from build123d import *

# Parameters (mm, degrees)
SKETCH1_R               = 45.95
BOSS_EXTRUDE1_DEPTH     = 3
SKETCH2_R               = 45.95
SKETCH2_R_2             = 40.95
BOSS_EXTRUDE2_DEPTH     = 22.4
SKETCH11_R              = 1.5
CUT_EXTRUDE1_DEPTH      = 46.95
CUT_EXTRUDE1_DEPTH_BACK = 46.95
SKETCH12_R              = 45.95
SKETCH12_R_2            = 40.95
BOSS_EXTRUDE3_DEPTH     = 25.4
SKETCH14_R              = 1.5
CUT_EXTRUDE2_DEPTH      = 46.95000011
CUT_EXTRUDE2_DEPTH_BACK = 46.95000011
SKETCH17_R              = 1.5
CUT_EXTRUDE4_DEPTH      = 10
SKETCH15_R              = 4
CUT_EXTRUDE6_DEPTH      = 10


with BuildPart() as part:
    # Sketch1 → Boss-Extrude1 (new body)
    with BuildSketch(Plane(origin=(0, 0, 0), x_dir=(1, 0, 0), z_dir=(0, 1, 0))):
        Circle(SKETCH1_R)
    extrude(amount=BOSS_EXTRUDE1_DEPTH)

    # Sketch2 → Boss-Extrude2 (add)
    with BuildSketch(Plane(origin=(0, 3, 0), x_dir=(1, 0, 0), z_dir=(0, 1, 0))):
        Circle(SKETCH2_R)
        Circle(SKETCH2_R_2, mode=Mode.SUBTRACT)
    extrude(amount=BOSS_EXTRUDE2_DEPTH)

    # Sketch11 → Cut-Extrude1 (cut, two sides)
    with BuildSketch(Plane.XY) as cut_extrude1_sk:
        with Locations((0, 13.9)):
            Circle(SKETCH11_R)
        with Locations((0, -13.9)):
            Circle(SKETCH11_R)
    extrude(amount=CUT_EXTRUDE1_DEPTH, mode=Mode.SUBTRACT)
    extrude(cut_extrude1_sk.sketch, amount=-CUT_EXTRUDE1_DEPTH_BACK, mode=Mode.SUBTRACT)

    # Sketch12 → Boss-Extrude3 (add)
    with BuildSketch(Plane(origin=(0, 25.4, 0), x_dir=(1, 0, 0), z_dir=(0, 1, 0))):
        Circle(SKETCH12_R)
        Circle(SKETCH12_R_2, mode=Mode.SUBTRACT)
    extrude(amount=BOSS_EXTRUDE3_DEPTH)

    # Sketch14 → Cut-Extrude2 (cut, two sides)
    with BuildSketch(Plane.XY) as cut_extrude2_sk:
        with Locations((0, 36.9)):
            Circle(SKETCH14_R)
    extrude(amount=CUT_EXTRUDE2_DEPTH, mode=Mode.SUBTRACT)
    extrude(cut_extrude2_sk.sketch, amount=-CUT_EXTRUDE2_DEPTH_BACK, mode=Mode.SUBTRACT)

    # Sketch17 → Cut-Extrude4 (cut)
    with BuildSketch(Plane(origin=(0, 3, 0), x_dir=(1, 0, 0), z_dir=(0, 1, 0))):
        with Locations((0, 9.5)):
            Circle(SKETCH17_R)
        with Locations((8.227241336, 4.75)):
            Circle(SKETCH17_R)
        with Locations((8.227241336, -4.75)):
            Circle(SKETCH17_R)
        with Locations((0, -9.5)):
            Circle(SKETCH17_R)
        with Locations((-8.227241336, -4.75)):
            Circle(SKETCH17_R)
        with Locations((-8.227241336, 4.75)):
            Circle(SKETCH17_R)
    extrude(amount=-CUT_EXTRUDE4_DEPTH, mode=Mode.SUBTRACT)

    # Sketch15 → Cut-Extrude6 (cut)
    with BuildSketch(Plane(origin=(0, 3, 0), x_dir=(1, 0, 0), z_dir=(0, 1, 0))):
        Circle(SKETCH15_R)
    extrude(amount=-CUT_EXTRUDE6_DEPTH, mode=Mode.SUBTRACT)


solid = part.part
Source: CAD feature listing. Evaluate the final solid. Frame: model axes, mm. A direction names the side the tool comes from. Give positions to 0.01 mm unless a question says otherwise; leave off trailing zeros. Order: outer loops, then holes, each group sorted by start corner. A loop starts at its lowest first (then second) coordinate and runs counter-clockwise, first axis right, second up. Notation, with made-up numbers: (-14, -26.5) -> (27, -26.5) arc R8 cw to (27, -15.5) -> close; hole circle Ø7 at (72.25, -33). An arc over 180 degrees is marked (long way). Use a Markdown table: item, result.
1) Section query A-A, the plane z = 0. Return the cut outline in (x, y).
Answer list:
| item | result |
|---|---|
| outline | (-45.95, 0) -> (-4, 0) -> (-4, 3) -> (-40.95, 3) -> (-40.95, 50.8) -> (-45.95, 50.8) -> close; (4, 0) -> (45.95, 0) -> (45.95, 50.8) -> (40.95, 50.8) -> (40.95, 3) -> (4, 3) -> close |
2) Ray query, line 1 along Z through (x, y) = (0, 2.25); line 2 along X through (y, z) = (19, 0); line 3 along Z through (x, y) = (-1.5, 32.5). Return the intervals inside material, ascending. Write a range as [from, to].
Answer list:
| item | result |
|---|---|
| line 1 | [-45.95, -11], [-8, -4], [4, 8], [11, 45.95] |
| line 2 | [-45.95, -40.95], [40.95, 45.95] |
| line 3 | [-45.93, -40.92], [40.92, 45.93] |
3) Mould query, pull axis Z, two halves, no side actions, for faces 1 (the cylindrical face through (9.613, 1.521, -4.175)), 2 (the flat face through (10, 0, -1)), 3 (the cylindrical face through (-9.961, 25.044, 44.857)). Classes: +Z half, -Z half, draft (parallel to the pull), parting line (faces both ways), or undercut.
Answer list:
| item | result |
|---|---|
| face 1 | undercut |
| face 2 | draft |
| face 3 | parting line |
4) Section query D-D, the plane z = -20.5. Return the cut outline in (x, y), then the cut area to 3 significant figures.
Answer list:
| item | result |
|---|---|
| outline | (-41.12, 0) -> (41.12, 0) -> (41.12, 50.8) -> (35.45, 50.8) -> (35.45, 3) -> (-35.45, 3) -> (-35.45, 50.8) -> (-41.12, 50.8) -> close |
| area | 789 mm² |
5) Contact query for flat-ended pins moving along their axis: P1, Ø5, axis at x = 0, z = -9.5, coming from the -Y side; P2, Ø3, axis at x = -22, z = 26.5, coming from the +Y side; P3, Ø4, axis at x = -24.5, y = 44, coming from the -Z side; P4, Ø1, axis at x = -1.5, y = 13.5, coming from the +Z side. Output: stop coordinate, or through.
Answer list:
| item | result |
|---|---|
| P1 | y = 0 |
| P2 | y = 3 |
| P3 | z = -40.06 |
| P4 | z = 45.93 |
6) Section query C-C, the plane x = 28.5. Return the cut outline in (y, z).
Answer list:
| item | result |
|---|---|
| outline | (0, -36.04) -> (50.8, -36.04) -> (50.8, -29.4) -> (3, -29.4) -> (3, 29.4) -> (50.8, 29.4) -> (50.8, 36.04) -> (0, 36.04) -> close |
7) Reachability of faces 4 (the cylindrical face through (-0.325, 35.436, -43.401)), 5 (the flat face through (9, 3, -1)) from +Z, -Z, +X, -X, +Y, -Y: full face, straight path, thin tool, end or side. Return the list, or none.
Answer list:
| item | result |
|---|---|
| face 4 | +Z, -Z |
| face 5 | +Y |
